```python
from build123d import *

# Parameters (mm, degrees)
F0_W      = 15
F0_H      = 15
F1_DEPTH  = 15
F2_W      = 10
F2_H      = 7
F3_DEPTH  = 8.5
F4_W      = 4
F4_H      = 7
F5_DEPTH  = 3
F6_W      = 4
F6_H      = 7
F7_DEPTH  = 3
F8_W      = 4
F8_H      = 2
F9_DEPTH  = 2
F10_W     = 4
F10_H     = 2
F11_DEPTH = 2
F12_W     = 14
F12_H     = 3
F13_DEPTH = 3
F14_W     = 14
F14_H     = 3
F15_DEPTH = 3
F16_W     = 5
F16_H     = 5
F17_DEPTH = 4
F18_W     = 15
F18_H     = 1
F19_DEPTH = 1
F20_W     = 1
F20_H     = 1
F21_DEPTH = 1
F22_W     = 1
F22_H     = 1
F23_DEPTH = 1
F24_W     = 2
F24_H     = 2
F25_DEPTH = 0.5
F26_W     = 2
F26_H     = 2
F27_DEPTH = 0.5
F28_W     = 2
F28_H     = 2
F29_DEPTH = 0.5
F30_W     = 10
F30_H     = 6.25
F31_DEPTH = 0.05
F32_W     = 2
F32_H     = 1
F33_DEPTH = 0.05
F34_W     = 1
F34_H     = 1
F35_DEPTH = 0.05
F36_W     = 7.05
F36_H     = 8.25
F37_DEPTH = 0.05
F38_W     = 1
F38_H     = 1
F39_DEPTH = 0.05
F40_W     = 7.1
F40_H     = 6.25
F41_DEPTH = 0.05


with BuildPart() as f1:
    # F0 (on Front) → F1 (new body)
    with BuildSketch(Plane.XZ):
        Rectangle(F0_W, F0_H)
    extrude(amount=F1_DEPTH)

    # F2 (on face) → F3 (join)
    with BuildSketch(Plane(origin=(0, 0, -7.5), x_dir=(1, 0, 0), z_dir=(0, 0, -1))):
        with Locations((0, 6.5)):
            Rectangle(F2_W, F2_H)
    extrude(amount=F3_DEPTH)

    # F4 (on face) → F5 (join)
    with BuildSketch(Plane(origin=(0, 0, -16), x_dir=(1, 0, 0), z_dir=(0, 0, -1))):
        with Locations((-3, 6.5)):
            Rectangle(F4_W, F4_H)
    extrude(amount=F5_DEPTH)

    # F6 (on face) → F7 (join)
    with BuildSketch(Plane(origin=(0, 0, -16), x_dir=(1, 0, 0), z_dir=(0, 0, -1))):
        with Locations((3, 6.5)):
            Rectangle(F6_W, F6_H)
    extrude(amount=F7_DEPTH)

    # F8 (on face) → F9 (join)
    with BuildSketch(Plane(origin=(0, -3, 0), x_dir=(-1, 0, 0), z_dir=(0, 1, 0))):
        with Locations((-3, -18)):
            Rectangle(F8_W, F8_H)
    extrude(amount=F9_DEPTH)

    # F10 (on face) → F11 (join, symmetric)
    with BuildSketch(Plane(origin=(0, -3, 0), x_dir=(-1, 0, 0), z_dir=(0, 1, 0))):
        with Locations((3, -18)):
            Rectangle(F10_W, F10_H)
    extrude(amount=F11_DEPTH, both=True)

    # F12 (on face) → F13 (join)
    with BuildSketch(Plane.YZ.offset(5)):
        with Locations((-2, -9)):
            Rectangle(F12_W, F12_H)
    extrude(amount=F13_DEPTH)

    # F14 (on face) → F15 (join)
    with BuildSketch(Plane(origin=(-5, 0, 0), x_dir=(0, -1, 0), z_dir=(-1, 0, 0))):
        with Locations((2, -9)):
            Rectangle(F14_W, F14_H)
    extrude(amount=F15_DEPTH)

    # F16 (on face) → F17 (join)
    with BuildSketch(Plane(origin=(0, 0, 0), x_dir=(-1, 0, 0), z_dir=(0, 1, 0))):
        with Locations((0, -5)):
            Rectangle(F16_W, F16_H)
    extrude(amount=F17_DEPTH)

    # F18 (on face) → F19 (join)
    with BuildSketch(Plane(origin=(0, 0, 0), x_dir=(-1, 0, 0), z_dir=(0, 1, 0))):
        with Locations((0, 2)):
            Rectangle(F18_W, F18_H)
    extrude(amount=F19_DEPTH)

    # F20 (on face) → F21 (cut)
    with BuildSketch(Plane(origin=(0, 0, 0), x_dir=(-1, 0, 0), z_dir=(0, 1, 0))):
        with Locations((3, -5)):
            Rectangle(F20_W, F20_H)
    extrude(amount=-F21_DEPTH, mode=Mode.SUBTRACT)

    # F22 (on face) → F23 (cut)
    with BuildSketch(Plane(origin=(0, 0, 0), x_dir=(-1, 0, 0), z_dir=(0, 1, 0))):
        with Locations((-3, -5)):
            Rectangle(F22_W, F22_H)
    extrude(amount=-F23_DEPTH, mode=Mode.SUBTRACT)

    # F24 (on face) → F25 (cut)
    with BuildSketch(Plane(origin=(0, 0, 0), x_dir=(-1, 0, 0), z_dir=(0, 1, 0))):
        with Locations((-6.5, 0.5)):
            Rectangle(F24_W, F24_H)
    extrude(amount=-F25_DEPTH, mode=Mode.SUBTRACT)

    # F26 (on face) → F27 (cut)
    with BuildSketch(Plane(origin=(0, 0, 0), x_dir=(-1, 0, 0), z_dir=(0, 1, 0))):
        with Locations((-4.5, 0.5)):
            Rectangle(F26_W, F26_H)
    extrude(amount=-F27_DEPTH, mode=Mode.SUBTRACT)

    # F28 (on face) → F29 (cut)
    with BuildSketch(Plane(origin=(0, 0, 0), x_dir=(-1, 0, 0), z_dir=(0, 1, 0))):
        with Locations((6.5, 0.5)):
            Rectangle(F28_W, F28_H)
        with Locations((4.5, 0.5)):
            Rectangle(F28_W, F28_H)
    extrude(amount=-F29_DEPTH, mode=Mode.SUBTRACT)

    # F30 (on face) → F31 (join)
    with BuildSketch(Plane(origin=(0, -3, 0), x_dir=(-1, 0, 0), z_dir=(0, 1, 0))):
        with Locations((0, -10.625)):
            Rectangle(F30_W, F30_H)
    extrude(amount=F31_DEPTH)

    # F32 (on face) → F33 (join)
    with BuildSketch(Plane(origin=(0, -3, 0), x_dir=(-1, 0, 0), z_dir=(0, 1, 0))):
        with Locations((4, -14.25)):
            Rectangle(F32_W, F32_H)
    extrude(amount=F33_DEPTH)

    # F34 (on face) → F35 (join)
    with BuildSketch(Plane(origin=(0, -3, 0), x_dir=(-1, 0, 0), z_dir=(0, 1, 0))):
        with Locations((4.5, -15.25)):
            Rectangle(F34_W, F34_H)
    extrude(amount=F35_DEPTH)

    # F36 (on face) → F37 (join)
    with BuildSketch(Plane(origin=(-5, 0, 0), x_dir=(0, -1, 0), z_dir=(-1, 0, 0))):
        with Locations((6.475, -11.625)):
            Rectangle(F36_W, F36_H)
    extrude(amount=F37_DEPTH)

    # F38 (on face) → F39 (join)
    with BuildSketch(Plane.XZ.offset(10)):
        Polygon((5, -13.75), (5, -7.5), (-5.05, -7.5), (-5.05, -13.75), (-3.05, -13.75), align=None)
        Polygon((-3.05, -13.75), (-5.05, -13.75), (-5.05, -14.75), (-4.05, -14.75), (-3.05, -14.75), align=None)
        with Locations((-4.55, -15.25)):
            Rectangle(F38_W, F38_H)
    extrude(amount=F39_DEPTH)

    # F40 (on face) → F41 (join)
    with BuildSketch(Plane.YZ.offset(5)):
        with Locations((-6.5, -10.625)):
            Rectangle(F40_W, F40_H)
    extrude(amount=F41_DEPTH)


solid = f1.part
```
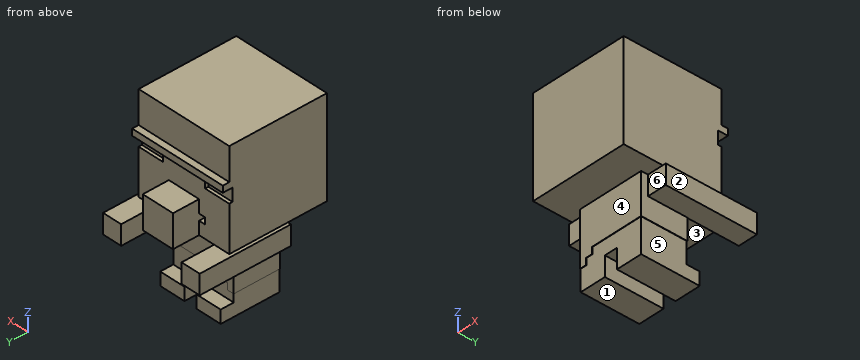
Design review of the part built by this model. Coordinates are the model's own, in mm. Face numbers are marked on the shaded views. A direction names the side the tool comes from. Coordinates: 2 decimals unless noted, no trailing zeros. Write each loop counter-clockwise with the first axis right and the second up, starting at its lowest first coordinate (ties: lowest second). Pieces come first, ordered by that corner, then holes.
1) To check wall thickness, follow L1, parallel to X at y = -7.5, z = -17.5; L2, parallel to Z at x = 6.5, y = 1.25; L3, parallel to X at y = -3.5, z = -13. State the ranges of each line that lie inside material, in increasing order.
2) Insertion check: pin 1 (0.9 mm diameter, centred on x = 6, y = -3, fed in from -Z); pin 2 (1.2 mm diameter, centred on x = 1, y = 2, fed in from +Z); pin 3 (2 mm diameter, centred on y = -13, z = 4, fed in from +X). Each pin has a flat end and moves straight along its axis. Give the tip position at first contact, or say it passes through.
3) Add section D-D (y = -7.5). Write out the cut boundary in (x, z), plus the area to 3 significant figures.
4) Mouldability with a two-part tool opening along Z and no side actions: class the marked faces 1, 2 and 3 as +Z half, -Z half, draft (parallel to the pull), parting line (faces both ways), or undercut.
5) Add section B-B (x = 2). Write out the cut boundary in (y, z).
6) Add section A-A (y = -2.25). Write out the cut boundary in (x, z).
7) Machinability: for the marked faces 4, 5 and 6, which of the approach directions +Z, -Z, +X, -X, +Y, -Y give a long, thin tool a straight path to every point of the face, cutting with its end or side? Answer none if there is none.
8) Add section C-C (z = -8.5). Write out the cut boundary in (x, y), plus the area to 3 significant figures.
Check result:
1. L1: x = -5 to -1, 1 to 5
1. L2: z = -10.5 to -7.5
1. L3: x = -5.05 to 5.05
2. pin 1: stops at z = -10.5
2. pin 2: stops at z = -2.5
2. pin 3: stops at x = 7.5
3. outline: (-8, -10.5) - (-5.05, -10.5) - (-5.05, -15.75) - (-5, -15.75) - (-5, -19) - (-1, -19) - (-1, -16) - (1, -16) - (1, -19) - (5, -19) - (5, -13.75) - (5.05, -13.75) - (5.05, -10.5) - (8, -10.5) - (8, -7.5) - (7.5, -7.5) - (7.5, 7.5) - (-7.5, 7.5) - (-7.5, -7.5) - (-8, -7.5) - close
3. area: 352 mm2
4. face 1: -Z half
4. face 2: draft
4. face 3: undercut
5. outline: (-15, -7.5) - (-10.05, -7.5) - (-10.05, -13.75) - (-10, -13.75) - (-10, -19) - (-1, -19) - (-1, -17) - (-3, -17) - (-3, -13.75) - (-2.95, -13.75) - (-2.95, -7.5) - (4, -7.5) - (4, -2.5) - (0, -2.5) - (0, 1.5) - (1, 1.5) - (1, 2.5) - (0, 2.5) - (0, 7.5) - (-15, 7.5) - close
6. outline: (-8, -10.5) - (-5, -10.5) - (-5, -7.5) - (5, -7.5) - (5, -10.5) - (8, -10.5) - (8, -7.5) - (7.5, -7.5) - (7.5, 7.5) - (-7.5, 7.5) - (-7.5, -7.5) - (-8, -7.5) - close; (-5, -19) - (-1, -19) - (-1, -17) - (-5, -17) - close; (1, -19) - (5, -19) - (5, -17) - (1, -17) - close
7. face 4: -Z, +X, -X, -Y
7. face 5: -Z, +X, +Y, -Y
7. face 6: -Z, +X, -Y
8. outline: (-8, -9) - (-5.05, -9) - (-5.05, -10.05) - (5.05, -10.05) - (5.05, -9) - (8, -9) - (8, 5) - (5, 5) - (5, -2.95) - (-5, -2.95) - (-5, 5) - (-8, 5) - close
8. area: 155 mm2
